Can you work these out from the model? Positions are in its coordinate system, mm. A direction names the side the tool comes from. Give positions to 0.01 mm unless a question says otherwise; leave off trailing zeros. Write each loop counter-clockwise with the first axis right and the second up, starting at its lowest first coordinate (ties: lowest second). Pieces come first, ordered by that corner, then holes.
1. Suppose I cut it at D-D (y = 7.5). Please give me the cut outline in (x, z).
2. On a 3-axis mill with a long thin cutter (end or side, diameter ignored), from which of +Z, -Z, +X, -X, +Y, -Y can I reach the whole of each face in a straight line? I mean faces 1 (the flat face through (2, 3, 0.864)), 2 (the flat face through (0.864, 3, -2)), 3 (the cylindrical face through (-0.653, 7.584, -0.852)), 4 (the flat face through (-0.864, 3, -2)). Say none if no direction works.
3. Suppose I cut it at C-C (z = 0). Please give me the cut outline in (x, y), and give its area (3 significant figures).
4. Suppose I cut it at B-B (x = 0). Please give me the cut outline in (y, z).
5. Suppose I cut it at A-A (y = 3.5). Please give me the cut outline in (x, z), and give its area (3 significant figures).
6. I'm going to push flat-ended pins straight in: pin 1 (0.5 mm diameter, centred on x = 0, z = 0.5, fed in from +Y); pin 2 (0.5 mm diameter, centred on x = 2, y = 2, fed in from +Z); pin 3 (1.2 mm diameter, centred on x = -1.5, y = 2.5, fed in from -Z). Where does each tip first touch, or does it pass through?
7. Thinking about a two-plate mould opening in Z: for faces 5 (the cylindrical face through (0.824, 5.653, -0.108)), 6 (the flat face through (0.864, 3, 2)), 7 (the flat face through (-2, 3, -0.864)), which applies, pulls with the +Z half, pulls with the -Z half, needs draft (parallel to the pull), parting line crosses it, or undercut?
8. If I drill on probe 1 along X at (y, z) = (4.75, 0); probe 2 along Z at (x, y) = (2, 4.25); probe 3 along Y at (x, z) = (-1.4, -0.35), over which ranges is the centre line in solid material (lowest first)?
```python
from build123d import *

# Parameters (mm, degrees)
BOSS_EXTRUDE1_DEPTH = 5.08
SKETCH2_R           = 1.073303583
SKETCH2_R_2         = 0.831378849
BOSS_EXTRUDE2_DEPTH = 5.08
CUT_EXTRUDE1_START  = -3.81
SKETCH4_R           = 0.831378849
CUT_EXTRUDE1_DEPTH  = 3.81


with BuildPart() as part:
    # Sketch1 → Boss-Extrude1 (new body)
    with BuildSketch(Plane(origin=(0, 0, 0), x_dir=(1, 0, 0), z_dir=(0, 1, 0))):
        Polygon((0.8636, 0.8636), (2.413, 0.8636), (2.413, -0.8636), (0.8636, -0.8636), (0.8636, -2.413), (-0.8636, -2.413), (-0.8636, -0.8636), (-2.413, -0.8636), (-2.413, 0.8636), (-0.8636, 0.8636), (-0.8636, 2.413), (0.8636, 2.413), align=None)
    extrude(amount=BOSS_EXTRUDE1_DEPTH)

    # Sketch2 → Boss-Extrude2 (add)
    with BuildSketch(Plane(origin=(0, 5.08, 0), x_dir=(1, 0, 0), z_dir=(0, 1, 0))):
        with Locations(Location((0, 0, 0), (0, 0, 270))):
            Circle(SKETCH2_R)
        with Locations(Location((0, 0, 0), (0, 0, 270))):
            Circle(SKETCH2_R_2, mode=Mode.SUBTRACT)
    extrude(amount=BOSS_EXTRUDE2_DEPTH)

    # Sketch4 → Cut-Extrude1 (cut)
    with BuildSketch(Plane(origin=(0, 5.08, 0), x_dir=(1, 0, 0), z_dir=(0, 1, 0)).offset(CUT_EXTRUDE1_START)):
        with Locations(Location((0, 0, 0), (0, 0, 270))):
            Circle(SKETCH4_R)
    extrude(amount=CUT_EXTRUDE1_DEPTH, mode=Mode.SUBTRACT)


solid = part.part
```
Checks:
1. outline: circle Ø2.15 at (0, 0); hole circle Ø1.66 at (0, 0)
2. face 1: +Z, +X, +Y, -Y
2. face 2: -Z, +X, +Y, -Y
2. face 3: +Y
2. face 4: -Z, -X, +Y, -Y
3. outline: (-2.41, 0) - (2.41, 0) - (2.41, 5.08) - (1.07, 5.08) - (1.07, 10.16) - (0.83, 10.16) - (0.83, 1.27) - (-0.83, 1.27) - (-0.83, 10.16) - (-1.07, 10.16) - (-1.07, 5.08) - (-2.41, 5.08) - close
3. area: 20.6 mm2
4. outline: (0, -2.41) - (5.08, -2.41) - (5.08, -1.07) - (10.16, -1.07) - (10.16, -0.83) - (1.27, -0.83) - (1.27, 0.83) - (10.16, 0.83) - (10.16, 1.07) - (5.08, 1.07) - (5.08, 2.41) - (0, 2.41) - close
5. outline: (-2.41, -0.86) - (-0.86, -0.86) - (-0.86, -2.41) - (0.86, -2.41) - (0.86, -0.86) - (2.41, -0.86) - (2.41, 0.86) - (0.86, 0.86) - (0.86, 2.41) - (-0.86, 2.41) - (-0.86, 0.86) - (-2.41, 0.86) - close; hole circle Ø1.66 at (0, 0)
5. area: 11.5 mm2
6. pin 1: stops at y = 1.27
6. pin 2: stops at z = 0.86
6. pin 3: stops at z = -0.86
7. face 5: undercut
7. face 6: needs draft
7. face 7: pulls with the -Z half
8. probe 1: x = -2.41 to -0.83, 0.83 to 2.41
8. probe 2: z = -0.86 to 0.86
8. probe 3: y = 0 to 5.08
